Design review of the part built by this model. Coordinates are the model's own, in mm. A direction names the side the tool comes from. Coordinates: 2 decimals unless noted, no trailing zeros. Loops run counter-clockwise (first coordinate to the right, second up) from the corner with the lowest first, then second, coordinate; pieces in that order, holes last. Notation, with made-up numbers: (43, 16.25) - (78, 16.25) arc R28 cw to (78, 46.25) - close; hole circle Ø4 at (-1.75, -7). An arc over 180 degrees is marked (long way). Use one line per item in the form item = value. Start each with the question number.
(1) Add section A-A (y = 0). State the section outline as (x, z) points.
(2) Clearance check with flat-ended pins moving along their axes: pin 1 Ø5 at (x, y) = (-5.48, 16.36) entering from -Z; pin 2 Ø1.3 at (x, z) = (-1, 6.5) entering from +Y; pin 3 Ø8 at (x, z) = (-4, 27) entering from -Y. State where each tip first meets the part, or that it passes through.
(3) Add section C-C (x = 0). State the section outline as (y, z) points, plus the area to 3 significant figures.
(4) For L1, parallel to Z at x = -24, y = 15; L2, parallel to X at y = -7, z = 30.5; L3, parallel to Y at x = -3, z = 4, list the stretches that pass through material, from the lowest coordinate up.
(5) Add section B-B (x = -18). State the section outline as (y, z) points.
(6) The part is to be moulded in two halves that separate along X. For faces 4 (the face through (28.14, 8.86, 31.48)), 5 (the face through (12.35, 11.15, 31.52)), 6 (the face through (0, 5.965, 5)), say which applies: pulls with the +X half, pulls with the -X half, needs draft (parallel to the pull), parting line crosses it, or undercut.
(7) Tool access review of faces 1 (the face through (-2.25, 5, 5)), 2 (the face through (0, 1, 0)), 3 (the face through (2.25, 5, 5)): name each direction out of +Z, -Z, +X, -X, +Y, -Y from which nothing blocks a thin tool from reaching the whole face with its end or side.
(8) Add section D-D (z = 22). State the section outline as (x, y) points, plus the area to 3 significant figures.
```python
from build123d import *

# Parameters (mm, degrees)
SKETCH_2_R          = 5
EXTRUDE_1_DEPTH     = 10
SKETCH_2_3_R        = 5
EXTRUDE_2_DEPTH     = 30
SKETCH_3_R          = 29.5
EXTRUDE_3_DEPTH     = 3
SKETCH_4_R          = 2
CUT_EXTRUDE_1_DEPTH = 3


with BuildPart() as part:
    # Sketch 2 → Extrude 1 (new body)
    with BuildSketch(Plane.XY):
        Circle(SKETCH_2_R)
        with BuildLine():
            Line((2.25, 5.965142775), (-2.25, 5.965142775))
            Line((-2.25, 5.965142775), (-2.25, 4.465142775))
            ThreePointArc((-2.25, 4.465142775), (0, 5), (2.25, 4.465142775))
            Line((2.25, 4.465142775), (2.25, 5.965142775))
        make_face()
    extrude(amount=EXTRUDE_1_DEPTH)

    # Sketch 2_3 → Extrude 2 (add)
    with BuildSketch(Plane.XY):
        with Locations(Location((0, 0, 0), (0, 0, 116.74368395))):
            Circle(SKETCH_2_3_R)
    extrude(amount=EXTRUDE_2_DEPTH)

    # Sketch 3 → Extrude 3 (add)
    with BuildSketch(Plane.XY.offset(30)):
        Circle(SKETCH_3_R)
    extrude(amount=EXTRUDE_3_DEPTH)

    # Sketch 4 → Cut-Extrude 1 (cut)
    with BuildSketch(Plane.XY.offset(33)):
        with Locations((-5.477961715, 16.357091289)):
            Circle(SKETCH_4_R)
        with Locations((11.426675731, 12.922599651)):
            Circle(SKETCH_4_R)
        with Locations((16.904637446, -3.434491638)):
            Circle(SKETCH_4_R)
        with Locations((5.477961715, -16.357091289)):
            Circle(SKETCH_4_R)
        with Locations((-11.426675731, -12.922599651)):
            Circle(SKETCH_4_R)
        with Locations((-16.904637446, 3.434491638)):
            Circle(SKETCH_4_R)
    extrude(amount=-CUT_EXTRUDE_1_DEPTH, mode=Mode.SUBTRACT)


solid = part.part
```
Computed values:
q1.outline = (-29.5, 30) - (-5, 30) - (-5, 0) - (5, 0) - (5, 30) - (29.5, 30) - (29.5, 33) - (-29.5, 33) - close
q2.pin_1 = 30
q2.pin_2 = 5.97
q2.pin_3 = -29.47
q3.outline = (-29.5, 30) - (-5, 30) - (-5, 0) - (5.97, 0) - (5.97, 10) - (5, 10) - (5, 30) - (29.5, 30) - (29.5, 33) - (-29.5, 33) - close
q3.area = 487 mm^2
q4.L1 = 30 to 33
q4.L2 = -28.66 to 28.66
q4.L3 = -4 to 4
q5.outline = (-23.37, 30) - (1.76, 30) - (1.76, 33) - (-23.37, 33) - close; (5.11, 30) - (23.37, 30) - (23.37, 33) - (5.11, 33) - close
q6.face_4 = parting line crosses it
q6.face_5 = undercut
q6.face_6 = needs draft
q7.face_1 = -Z, -X, +Y
q7.face_2 = -Z, +X, -X, +Y, -Y
q7.face_3 = -Z, +X, +Y
q8.outline = circle Ø10 at (0, 0)
q8.area = 78.5 mm^2
